Source: CAD feature listing. Evaluate the final solid. Frame: model axes, mm. Face numbers are marked on the shaded views. A direction names the side the tool comes from. Coordinates: 2 decimals unless noted, no trailing zeros. Write each loop counter-clockwise with the first axis right and the second up, starting at its lowest first coordinate (ties: lowest second). Pieces come first, ordered by that corner, then holes. Notation, with made-up numbers: (2, 25) - (18, 25) arc R13 cw to (18, 38) - close; hole circle Ø5 at (65.25, 9). An arc over 180 degrees is marked (long way). One line per question, with ' | ' between items.
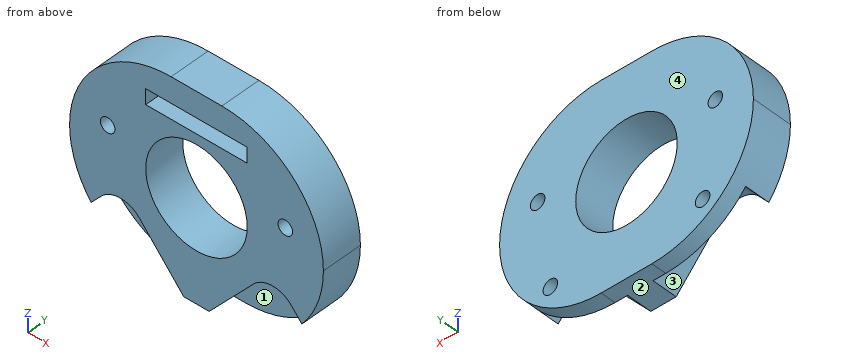
from build123d import *

# Parameters (mm, degrees)
PAD005_DEPTH    = 8
SKETCH018_W     = 20
SKETCH018_H     = 3
POCKET011_DEPTH = 5
SKETCH019_R     = 10
SKETCH019_R_2   = 1.43
POCKET012_DEPTH = 10


with BuildPart() as part:
    # Sketch017 → Pad005 (new body)
    with BuildSketch(Plane.XZ):
        with BuildLine():
            Line((-4.99996, 20), (4.99996, 20))
            ThreePointArc((25, 0), (19.142122, 14.14215), (4.99996, 20))
            ThreePointArc((4.99996, -20), (19.142122, -14.14215), (25, 0))
            Line((4.99996, -20), (-4.99996, -20))
            ThreePointArc((-25, 0), (-19.142122, -14.14215), (-4.99996, -20))
            ThreePointArc((-4.99996, 20), (-19.142122, 14.14215), (-25, 0))
        make_face()
    extrude(amount=PAD005_DEPTH)

    # Sketch018 (on Face8 of Pad005) → Pocket011 (cut)
    with BuildSketch(Plane.XZ.offset(8)):
        with BuildLine():
            ThreePointArc((-11.241388, -10.035935), (-15, -8.333333), (-18.758612, -10.035935))
            Line((-18.758612, -10.035935), (-27.5, -20))
            ThreePointArc((-27.5, -20), (-15, -47.594619), (-2.5, -20))
            Line((-2.5, -20), (-11.241388, -10.035935))
        make_face()
        with BuildLine():
            ThreePointArc((18.758612, -10.035935), (15, -8.333333), (11.241388, -10.035935))
            Line((11.241388, -10.035935), (2.5, -20))
            ThreePointArc((2.5, -20), (15, -47.594619), (27.5, -20))
            Line((27.5, -20), (18.758612, -10.035935))
        make_face()
        with Locations((0, 13.5)):
            Rectangle(SKETCH018_W, SKETCH018_H)
    extrude(amount=-POCKET011_DEPTH, mode=Mode.SUBTRACT)

    # Sketch019 (on Face5 of Pocket011) → Pocket012 (cut)
    with BuildSketch(Plane.XZ.offset(8)):
        Circle(SKETCH019_R)
        with Locations((-15, -13.333333)):
            Circle(SKETCH019_R_2)
        with Locations((15, -13.333333)):
            Circle(SKETCH019_R_2)
        with Locations((-17.5, 4)):
            Circle(SKETCH019_R_2)
        with Locations((17.5, 4)):
            Circle(SKETCH019_R_2)
    extrude(amount=-POCKET012_DEPTH, mode=Mode.SUBTRACT)


with BuildPart() as part_1:
    # Body005 placement: moved
    add(part.part.moved(Location((60, 55.5, 76.5))))


solid = part_1.part
Item 1: Pin query (flat end, axial travel): pin 1 Ø2.5 at (x, z) = (45, 63.17) entering from -Y; pin 2 Ø3.5 at (x, z) = (75, 63.17) entering from -Y; pin 3 Ø3.5 at (y, z) = (50, 89.5) entering from +X; pin 4 Ø4 at (x, y) = (40, 48.5) entering from -Z. Return the tip coordinate at first contact, or that it passes through.
Check sheet entries:
pin 1: through | pin 2: y = 52.5 | pin 3: x = 81.54 | pin 4: z = 64.18
Item 2: Ray query, line 1 along Z through (x, y) = (60.5, 50.5); line 2 along X through (y, z) = (51, 80.5); line 3 along Z through (x, y) = (61, 49). Return the intervals inside material, ascending. Write a range as [from, to].
Check sheet entries:
line 1: [56.5, 66.51], [86.49, 88.5], [91.5, 96.5] | line 2: [35.4, 41.07], [43.93, 50.83], [69.17, 76.07], [78.93, 84.6] | line 3: [56.5, 66.55], [86.45, 88.5], [91.5, 96.5]
Item 3: Cut plane A-A on x = 60. Return loops of the section in (y, z).
Check sheet entries:
outline: (47.5, 56.5) - (55.5, 56.5) - (55.5, 66.5) - (47.5, 66.5) - close; (47.5, 86.5) - (55.5, 86.5) - (55.5, 96.5) - (47.5, 96.5) - (47.5, 91.5) - (52.5, 91.5) - (52.5, 88.5) - (47.5, 88.5) - close
Item 4: Cut plane B-B on z = 85.5. Return loops of the section in (x, y).
Check sheet entries:
outline: (37.14, 47.5) - (55.64, 47.5) - (55.64, 55.5) - (37.14, 55.5) - close; (64.36, 47.5) - (82.86, 47.5) - (82.86, 55.5) - (64.36, 55.5) - close
Item 5: Mould query, pull axis X, two halves, no side actions, for the marked faces 1 and 2. Classes: pulls with the +X half, pulls with the -X half, needs draft (parallel to the pull), parting line crosses it, or undercut.
Check sheet entries:
face 1: undercut | face 2: needs draft
Item 6: Access query for the marked faces 3 and 4. Directions: +Z, -Z, +X, -X, +Y, -Y. A direction counts if a zero-diameter tool reaches every point of the face in a straight line with its end or side. Return the directions, or none.
Check sheet entries:
face 3: -Z, -Y | face 4: +Z, -Z, +X, -X, +Y
Item 7: Cut plane D-D on y = 53.25. Return loops of the section in (x, z), and give its area (3 significant figures).
Check sheet entries:
outline: (35, 76.5) arc R20 ccw to (55, 56.5) - (65, 56.5) arc R20 ccw to (85, 76.5) arc R20 ccw to (65, 96.5) - (55, 96.5) arc R20 ccw to start; hole circle Ø2.86 at (42.5, 80.5); hole circle Ø2.86 at (45, 63.17); hole circle Ø20 at (60, 76.5); hole circle Ø2.86 at (75, 63.17); hole circle Ø2.86 at (77.5, 80.5) | area: 1,320 mm²
Item 8: Cut plane C-C on y = 48.75. Return loops of the section in (x, z), and give its area (3 significant figures).
Check sheet entries:
outline: (35, 76.5) arc R20 ccw to (39.24, 64.18) - (41.24, 66.46) arc R5 cw to (48.76, 66.46) - (57.5, 56.5) - (62.5, 56.5) - (71.24, 66.46) arc R5 cw to (78.76, 66.46) - (80.76, 64.18) arc R20 ccw to (85, 76.5) arc R20 ccw to (65, 96.5) - (55, 96.5) arc R20 ccw to start; hole circle Ø2.86 at (42.5, 80.5); hole circle Ø20 at (60, 76.5); hole (50, 88.5) - (70, 88.5) - (70, 91.5) - (50, 91.5) - close; hole circle Ø2.86 at (77.5, 80.5) | area: 1,050 mm²
